from build123d import *

# Parameters (mm, degrees)
F0_W     = 62.237114
F0_H     = 55.183612
F1_DEPTH = 127
F2_R     = 15.198366
F3_DEPTH = 127
F5_DEPTH = 25.4


with BuildPart() as f1:
    # F0 (on Front) → F1 (new body)
    with BuildSketch(Plane.XZ):
        with Locations((31.118557, 27.591806)):
            Rectangle(F0_W, F0_H)
    extrude(amount=F1_DEPTH)

    # F2 (on face) → F3 (cut)
    with BuildSketch(Plane.XZ.offset(127)):
        with Locations((31.334992, 27.2323)):
            Circle(F2_R)
    extrude(amount=-F3_DEPTH, mode=Mode.SUBTRACT)

    # F4 (on face) → F5 (cut)
    with BuildSketch(Plane.XY.offset(55.183612)):
        Polygon((44.284318, -31.432733), (25.63932, -26.329752), (14.235882, -40.970355), (27.033182, -50.93806), (16.672973, -64.239287), (44.284318, -64.239287), align=None)
    extrude(amount=-F5_DEPTH, mode=Mode.SUBTRACT)


solid = f1.part
Could you check a few things on this model? Use its own coordinates, in mm. A direction names the side the tool comes from. Coordinates: 2 decimals unless noted, no trailing zeros. Write each loop counter-clockwise with the first axis right and the second up, starting at its lowest first coordinate (ties: lowest second). Pieces come first, ordered by that corner, then holes. Notation, with made-up numbers: (-9, 62.5) - (35, 62.5) arc R15 cw to (35, 82.5) - close; hole circle Ø9 at (26, -23.75). An arc over 180 degrees is marked (long way). Write item = value, one per line.
1) Suppose I cut it at C-C on y = -112. Please give me the cut outline in (x, z) (3 decimals), plus the area to 3 significant figures.
Result set:
outline = (0, 0) - (62.237, 0) - (62.237, 55.184) - (0, 55.184) - close; hole circle Ø30.397 at (31.335, 27.232)
area = 2,710 mm2
2) Suppose I cut it at A-A on z = 21. Please give me the cut outline in (x, y), plus the area to 3 significant figures.
Result set:
outline = (0, -127) - (17.47, -127) - (17.47, 0) - (0, 0) - close; (45.2, -127) - (62.24, -127) - (62.24, 0) - (45.2, 0) - close
area = 4,380 mm2
3) Suppose I cut it at D-D on x = 22. Please give me the cut outline in (y, z).
Result set:
outline = (-127, 0) - (0, 0) - (0, 15.24) - (-127, 15.24) - close; (-127, 39.23) - (-64.24, 39.23) - (-64.24, 55.18) - (-127, 55.18) - close; (-57.4, 39.23) - (-47.02, 39.23) - (-47.02, 55.18) - (-57.4, 55.18) - close; (-31, 39.23) - (0, 39.23) - (0, 55.18) - (-31, 55.18) - close
4) We'd pull the mould along Y, two halves only. Please class faces 1 (the flat face through (44.284, -48, 45)), 2 (the flat face through (31, -63, 0)), 3 (the flat face through (16.9, -127, 21.8)): +Y half, -Y half, draft (parallel to the pull), parting line (faces both ways), or undercut.
Result set:
face_1 = undercut
face_2 = draft
face_3 = -Y half
5) For faces 4 (the flat face through (18.75, -35.174, 45.484)), 5 (the cylindrical face through (28.04, -64.389, 12.395)), which set-ups out of +Z, -Z, +X, -X, +Y, -Y let a thin tool reach every point of the face, with its end or its side?
Result set:
face_4 = +Z
face_5 = +Y, -Y
6) Please list where these lines run through material, in increasing order: line 1 (X direction, y = -90, z = 14.5); line 2 (X direction, y = -110, z = 14); line 3 (Z direction, x = 34.5, y = -117.5). Write a range as [from, to].
Result set:
line_1 = [0, 23.04], [39.63, 62.24]
line_2 = [0, 23.86], [38.81, 62.24]
line_3 = [0, 12.37], [42.1, 55.18]
7) Suppose I cut it at B-B on x = 31.5. Please give me the cut outline in (y, z), plus the area to 3 significant figures.
Result set:
outline = (-127, 0) - (0, 0) - (0, 12.03) - (-127, 12.03) - close; (-127, 42.43) - (-64.24, 42.43) - (-64.24, 55.18) - (-127, 55.18) - close; (-27.93, 42.43) - (0, 42.43) - (0, 55.18) - (-27.93, 55.18) - close
area = 2,690 mm2
8) Will this pin go through, and if not, where does the flat tip stop? pin 1 Ø0.6 at (x, y) = (15, -41) entering from +Z.
Result set:
pin_1 = 29.78
